```python
from build123d import *


with BuildPart() as part:
    # Sketch → Revolution (revolve)
    with BuildSketch(Plane.XZ):
        with BuildLine():
            ThreePointArc((-10.790142, 0.3), (-10.702274, 0.087868), (-10.490142, 0))
            Line((-10.490142, 0), (-9.690142, 0))
            ThreePointArc((-9.690142, 0), (-9.47801, 0.087868), (-9.390142, 0.3))
            Line((-9.390142, 0.3), (-9.390142, 3.7))
            ThreePointArc((-9.390142, 3.7), (-9.47801, 3.912132), (-9.690142, 4))
            Line((-9.690142, 4), (-10.490142, 4))
            ThreePointArc((-10.490142, 4), (-10.702274, 3.912132), (-10.790142, 3.7))
            Line((-10.790142, 3.7), (-10.790142, 0.3))
        make_face()
    revolve(axis=Axis((0, 0, 0), (0, 0, 1)))


solid = part.part
```
Model file for the job. Use its own axes, mm. Give positions to 0.01 mm unless a question says otherwise; leave off trailing zeros. Write each loop counter-clockwise with the first axis right and the second up, starting at its lowest first coordinate (ties: lowest second). Pieces come first, ordered by that corner, then holes. Notation, with made-up numbers: (70, -14.5) -> (107, -14.5) arc R22 cw to (107, -1.5) -> close; hole circle Ø9 at (36.25, 28). An arc over 180 degrees is marked (long way). Use CSV: the item, a comma, the result in double quotes. Start each with the question number.
1) Drill centre lines: L1, parallel to X at y = 0, z = 2.75; L2, parallel to Y at x = 3.5, z = 2. Where is each one in solid material? Low to high.
2) Cut at A-A on x = 0. List the corners of the cut face in (y, z).
3) Pin check, flat tip, straight feed: P1, Ø1, axis at x = -1.5, z = 1.5, coming from the -Y side. Stop position of the tip, or through.
4) Cut at C-C on z = 1.5. List the corners of the cut face in (x, y), plus the area to 3 significant figures.
5) Two-plate mould, pull along X, no slides. Class faces 1 (the cylindrical face through (2.339, 10.534, 1.976)), 2 (the flat face through (7, 7, 4)), 3 (the cylindrical face through (7.452, 5.714, 2.024)): released by +X, released by -X, zero draft, split by the parting line, or undercut.
Final values:
1,L1,"x = -10.79 to -9.39, 9.39 to 10.79"
1,L2,"y = -10.21 to -8.71, 8.71 to 10.21"
2,outline,"(-10.79, 0.3) arc R0.3 ccw to (-10.49, 0) -> (-9.69, 0) arc R0.3 ccw to (-9.39, 0.3) -> (-9.39, 3.7) arc R0.3 ccw to (-9.69, 4) -> (-10.49, 4) arc R0.3 ccw to (-10.79, 3.7) -> close; (9.39, 0.3) arc R0.3 ccw to (9.69, 0) -> (10.49, 0) arc R0.3 ccw to (10.79, 0.3) -> (10.79, 3.7) arc R0.3 ccw to (10.49, 4) -> (9.69, 4) arc R0.3 ccw to (9.39, 3.7) -> close"
3,P1,"stops at y = -10.74"
4,outline,"circle Ø21.58 at (0, 0); hole circle Ø18.78 at (0, 0)"
4,area,"88.8 mm2"
5,face 1,"split by the parting line"
5,face 2,"zero draft"
5,face 3,"undercut"
